Source: CAD feature listing. Evaluate the final solid. Frame: model axes, mm. Coordinates: 2 decimals unless noted, no trailing zeros. Loops run counter-clockwise (first coordinate to the right, second up) from the corner with the lowest first, then second, coordinate; pieces in that order, holes last.
```python
from build123d import *

# Parameters (mm, degrees)
SKETCH1_R           = 2.5
BOSS_EXTRUDE1_DEPTH = 6
SKETCH2_W           = 10
SKETCH2_H           = 6
SKETCH2_W_2         = 6
SKETCH2_H_2         = 10
CUT_EXTRUDE1_DEPTH  = 134.97761007
SKETCH3_R           = 1.5
CUT_EXTRUDE2_DEPTH  = 134.97761007
CAVITY1_OUTLINE_R   = 1.5
CAVITY1_DEPTH       = 6


# Read off the part's stored shape, not the designer's step: Cavity1
with BuildPart() as part:
    # Sketch1 → Boss-Extrude1 (new body)
    with BuildSketch(Plane.XY):
        with BuildLine():
            Line((-9.685424338, 2.488484559), (5.386220056, 61.148792841))
            ThreePointArc((5.386220056, 61.148792841), (15.733633721, 76.897010412), (33.561388608, 83))
            Line((33.561388608, 83), (105, 83))
            Line((105, 83), (105, 0))
            Line((105, 0), (-10.324792855, 0))
            Line((-10.324792855, 0), (-9.685424338, 2.488484559))
        make_face()
        with Locations((33.561388608, 53.909722104)):
            Circle(SKETCH1_R, mode=Mode.SUBTRACT)
    extrude(amount=BOSS_EXTRUDE1_DEPTH)

    # Sketch2 → Cut-Extrude1 (cut, through all)
    with BuildSketch(Plane.XY.offset(6)):
        with Locations((15, 3)):
            Rectangle(SKETCH2_W, SKETCH2_H)
        with Locations((57.5, 3)):
            Rectangle(SKETCH2_W, SKETCH2_H)
        with Locations((100, 3)):
            Rectangle(SKETCH2_W, SKETCH2_H)
        with Locations((102, 19.75)):
            Rectangle(SKETCH2_W_2, SKETCH2_H_2)
        with Locations((13, 19.75)):
            Rectangle(SKETCH2_W_2, SKETCH2_H_2)
    extrude(amount=-CUT_EXTRUDE1_DEPTH, mode=Mode.SUBTRACT)

    # Sketch3 → Cut-Extrude2 (cut, through all)
    with BuildSketch(Plane.XY.offset(6)):
        with Locations((50, 78)):
            Circle(SKETCH3_R)
        with Locations((100, 78)):
            Circle(SKETCH3_R)
    extrude(amount=-CUT_EXTRUDE2_DEPTH, mode=Mode.SUBTRACT)

    # Cavity1 outline → Cavity1 (cut)
    with BuildSketch(Plane.XY):
        with Locations((8.414860226, 52.844005614)):
            Circle(CAVITY1_OUTLINE_R)
    extrude(amount=CAVITY1_DEPTH, mode=Mode.SUBTRACT)


solid = part.part
```
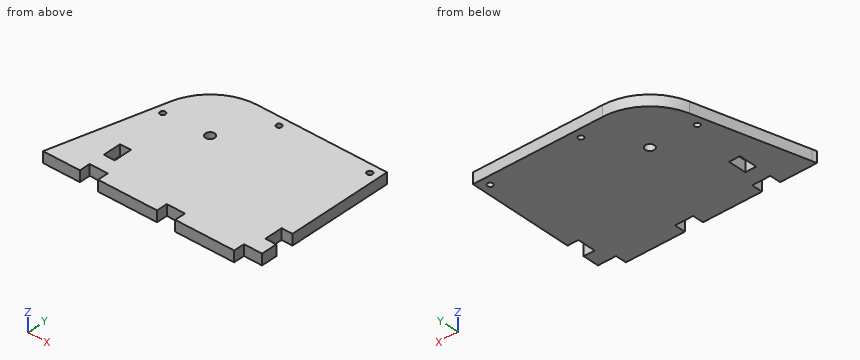
Q1. Section query C-C on y = 78. Return the cut outline in (x, z).
Q2. Material intervals for line 1 along Y through (x, z) = (100, 3.45); line 2 along X through (y, z) = (78, 1.55); line 3 along Y through (x, z) = (33.5, 2), sorted ascending.
Q3. Section query B-B on y = 16. Return the cut outline in (x, z), then the cut area to 3 significant figures.
Q4. First-contact query: pin 1 Ø3 at (x, z) = (102, 1.5) entering from -Y; pin 2 Ø3 at (x, z) = (20, 3) entering from -Y; pin 3 Ø2.5 at (x, y) = (8.41, 52.84) entering from -Z; pin 4 Ø1.8 at (y, z) = (21.5, 3.5) entering from -X. Flat tips, straight axial feed; report the tip coordinate or a pass-through.
Q5. Section query A-A on x = 50. Return the cut outline in (y, z).
Q6. Section query D-D on z = 3.8. Return the cut outline in (x, y).
Resolved:
1. outline: (17.25, 0) - (48.5, 0) - (48.5, 6) - (17.25, 6) - close; (51.5, 0) - (98.5, 0) - (98.5, 6) - (51.5, 6) - close; (101.5, 0) - (105, 0) - (105, 6) - (101.5, 6) - close
2. line 1: y = 6 to 14.75, 24.75 to 76.5, 79.5 to 83
2. line 2: x = 17.25 to 48.5, 51.5 to 98.5, 101.5 to 105
2. line 3: y = 0 to 51.41, 56.41 to 83
3. outline: (-6.21, 0) - (10, 0) - (10, 6) - (-6.21, 6) - close; (16, 0) - (99, 0) - (99, 6) - (16, 6) - close
3. area: 595 mm2
4. pin 1: stops at y = 6
4. pin 2: stops at y = 0
4. pin 3: passes through
4. pin 4: stops at x = -5.03
5. outline: (0, 0) - (76.5, 0) - (76.5, 6) - (0, 6) - close; (79.5, 0) - (83, 0) - (83, 6) - (79.5, 6) - close
6. outline: (-10.32, 0) - (10, 0) - (10, 6) - (20, 6) - (20, 0) - (52.5, 0) - (52.5, 6) - (62.5, 6) - (62.5, 0) - (95, 0) - (95, 6) - (105, 6) - (105, 14.75) - (99, 14.75) - (99, 24.75) - (105, 24.75) - (105, 83) - (33.56, 83) arc R29.09 ccw to (5.39, 61.15) - close; hole circle Ø3 at (8.41, 52.84); hole (10, 14.75) - (16, 14.75) - (16, 24.75) - (10, 24.75) - close; hole circle Ø5 at (33.56, 53.91); hole circle Ø3 at (50, 78); hole circle Ø3 at (100, 78)
